Model file for the job. Use its own axes, mm. A direction names the side the tool comes from. Give positions to 0.01 mm unless a question says otherwise; leave off trailing zeros. Loops run counter-clockwise (first coordinate to the right, second up) from the corner with the lowest first, then second, coordinate; pieces in that order, holes last. Notation, with made-up numbers: (73, -13.5) - (115, -13.5) arc R21 ccw to (115, -4.5) - close; hole circle Ø5 at (57, 30.5). An arc over 180 degrees is marked (long way). Answer as CSV lines item,"result". Start each with the question number.
Item 1: Saw through at A-A on y = 0. Give the cut face in (x, z), plus the area to 3 significant figures.
Item 2: Saw through at B-B on x = -12. Give the cut face in (y, z), plus the area to 3 significant figures.
Item 3: Pull direction Z, two halves, no side cores. Call faces 4 (the flat face through (-0.15, 17.96, 25.19)), 5 (the cylindrical face through (-35.294, 0.028, 27.434)), 6 (the flat face through (11, 0, 15)): pulls with the +Z half, pulls with the -Z half, needs draft (parallel to the pull), parting line crosses it, or undercut.
Item 4: Tool access for faces 1 (the flat face through (-17.5, 7, 26)), 2 (the flat face through (-0.154, -16.768, 21.258)), 3 (the flat face through (-0.15, -14.12, 22.89)): list every direction of +Z, -Z, +X, -X, +Y, -Y with a clear straight run to the whole face (end or side of a thin tool).
Item 5: Saw through at C-C on y = -25. Give the cut face in (x, z).
Item 6: Drill centre lines: L1, parallel to Y at x = -16.5, z = 24; L2, parallel to Z at x = -19, y = 4; L3, parallel to Y at x = -30, z = 8. Where is each one in solid material? Low to high. Write a range as from..to.
Item 7: Pin check, flat tips, straight feed: pin 1 (2 mm diameter, centred on x = -14, z = 18, fed in from +Y); pin 2 (5 mm diameter, centred on y = 7, z = 18.5, fed in from -X); pin 3 (2.5 mm diameter, centred on x = -32, z = 9, fed in from +Y) (3 decimals); pin 4 (3.5 mm diameter, centred on x = -19, z = 21, fed in from -Y). Stop position of each tip, or through.
Item 8: Saw through at D-D on z = 4. Give the cut face in (x, y), plus the area to 3 significant figures.
from build123d import *

# Parameters (mm, degrees)
ESBO_O2_R                  = 7.6
ESBO_O2_W                  = 7
ESBO_O2_H                  = 10
RESSALTO_EXTRUS_O1_DEPTH   = 30
CORTE_EXTRUS_O1_DEPTH      = 52.819397912
CORTE_EXTRUS_O2_DEPTH      = 68.825142831
CORTE_EXTRUS_O2_DEPTH_BACK = 68.825142831
ESBO_O4_R                  = 1.6
FILETE2_R                  = 9
CORTE_EXTRUS_O3_DEPTH      = 67.882564304
CORTE_EXTRUS_O3_DEPTH_BACK = 10
ESBO_O7_R                  = 1.6


with BuildPart() as part:
    # Esboço2 → Ressalto-extrusão1 (new body)
    with BuildSketch(Plane.XY):
        Polygon((-11, 15), (-11, 32.5), (11, 32.5), (11, -32.5), (-11, -32.5), (-11, -15), (-26.5, -15), (-26.5, -12), (-10.5, -12), (-10.5, -2), (-26.5, -2), (-38, -2), (-38, 2), (-22, 2), (-22, 12), (-38, 12), (-38, 15), align=None)
        Circle(ESBO_O2_R, mode=Mode.SUBTRACT)
        with Locations((-14, 7)):
            Rectangle(ESBO_O2_W, ESBO_O2_H, mode=Mode.SUBTRACT)
    extrude(amount=RESSALTO_EXTRUS_O1_DEPTH)

    # Esboço3 → Corte-extrusão1 (cut, through all)
    with BuildSketch(Plane.ZY.offset(11)):
        Polygon((30, 26.434795421), (19.494757511, 32.5), (30, 32.5), align=None)
        Polygon((18.952178178, 18.099406712), (23.628715358, 15.399406712), (22.128715358, 12.8013305), (17.452178178, 15.5013305), align=None)
        with BuildLine():
            Line((17.854101966, 22.197482923), (31.133039027, 14.530885036))
            Line((31.133039027, 14.530885036), (32.133039027, 16.262935844))
            Line((32.133039027, 16.262935844), (18.854101966, 23.929533731))
            ThreePointArc((18.854101966, 23.929533731), (11.535898385, 27), (17.854101966, 22.197482923))
        make_face()
        with BuildLine():
            Line((31.133039027, -14.530885036), (32.133039027, -16.262935844))
            Line((32.133039027, -16.262935844), (18.854101966, -23.929533731))
            ThreePointArc((18.854101966, -23.929533731), (11.535898385, -27), (17.854101966, -22.197482923))
            Line((17.854101966, -22.197482923), (31.133039027, -14.530885036))
        make_face()
        Polygon((23.628715358, -15.399406712), (22.128715358, -12.8013305), (17.452178178, -15.5013305), (18.952178178, -18.099406712), align=None)
        Polygon((0, 26.434795421), (10.505242489, 32.5), (0, 32.5), align=None)
        Polygon((30, -32.5), (19.494757511, -32.5), (30, -26.434795421), align=None)
        Polygon((0, -32.5), (10.505242489, -32.5), (0, -26.434795421), align=None)
    extrude(amount=-CORTE_EXTRUS_O1_DEPTH, mode=Mode.SUBTRACT)

    # Esboço4 → Corte-extrusão2 (cut, two sides: drawn at the far end of the back side and taken through both)
    with BuildSketch(Plane(origin=(0, 15, 0), x_dir=(1, 0, 0), z_dir=(0, 1, 0)).offset(-CORTE_EXTRUS_O2_DEPTH_BACK)):
        with Locations(Location((-32, -9, 0), (0, 0, 270))):
            Circle(ESBO_O4_R)
        with Locations(Location((-19, -21, 0), (0, 0, 270))):
            Circle(ESBO_O4_R)
    extrude(amount=CORTE_EXTRUS_O2_DEPTH + CORTE_EXTRUS_O2_DEPTH_BACK, mode=Mode.SUBTRACT)

    # Filete2
    filete2_edges = [part.edges().sort_by_distance(p)[0] for p in [
        (-38, 13.5, 30),
        (-26.5, -13.5, 0),
        (-38, 0, 0),
        (-38, 13.5, 0),
        (-38, 0, 30),
        (-26.5, -13.5, 30),
    ]]
    fillet(filete2_edges, radius=FILETE2_R)

    # Esboço7 → Corte-extrusão3 (cut, two sides: drawn at the far end of the back side and taken through both)
    with BuildSketch(Plane(origin=(0, 19.183012702, 11.075317547), x_dir=(1, 0, 0), z_dir=(0, 0.8660254037844418, 0.4999999999999945)).offset(-CORTE_EXTRUS_O3_DEPTH_BACK)):
        with Locations(Location((0, -10.063364403, 0), (0, 0, 90))):
            Circle(ESBO_O7_R)
    extrude(amount=CORTE_EXTRUS_O3_DEPTH + CORTE_EXTRUS_O3_DEPTH_BACK, mode=Mode.SUBTRACT)


solid = part.part
Responses:
1,outline,"(-38, 9) arc R9 ccw to (-29, 0) - (-7.6, 0) - (-7.6, 30) - (-29, 30) arc R9 ccw to (-38, 21) - close; (7.6, 0) - (11, 0) - (11, 30) - (7.6, 30) - close; hole circle Ø3.2 at (-32, 9); hole circle Ø3.2 at (-19, 21)"
1,area,"963 mm2"
2,outline,"(-15, 0) - (-12, 0) - (-12, 30) - (-15, 30) - close; (-2, 0) - (2, 0) - (2, 30) - (-2, 30) - close; (12, 0) - (15, 0) - (15, 30) - (12, 30) - close"
2,area,"300 mm2"
3,face 4,"undercut"
3,face 5,"pulls with the +Z half"
3,face 6,"needs draft"
4,face 1,"+Z, -Z"
4,face 2,"+X, -X"
4,face 3,"+X"
5,outline,"(-11, 0) - (11, 0) - (11, 11) - (-11, 11) - close; (-11, 19) - (11, 19) - (11, 30) - (-11, 30) - close"
6,L1,"-15..-12, -2..2, 12..15"
6,L2,"0..19.4, 22.6..30"
6,L3,"-2..2, 12..15"
7,pin 1,"y = 15"
7,pin 2,"x = -22"
7,pin 3,"through"
7,pin 4,"y = -15"
8,outline,"(-36.48, -2) - (-10.5, -2) - (-10.5, -12) - (-24.98, -12) - (-24.98, -15) - (-11, -15) - (-11, -28.74) - (11, -28.74) - (11, 28.74) - (-11, 28.74) - (-11, 15) - (-36.48, 15) - (-36.48, 12) - (-22, 12) - (-22, 2) - (-36.48, 2) - close; hole (-17.5, 2) - (-10.5, 2) - (-10.5, 12) - (-17.5, 12) - close; hole circle Ø15.2 at (0, 0)"
8,area,"1,340 mm2"
